Can you work these out from the drawing? Everything is in mm from the part's minimum corner. Round coordinates to 2 decimals unless told otherwise and drop trailing zeros. Order: outer loops, then holes, each group sorted by start corner. A loop starts at its lowest first (then second) coordinate and runs counter-clockwise, first axis right, second up. Notation, with made-up numbers: (89, 67.25) - (141, 67.25) arc R19 cw to (141, 72.25) - close; hole circle Ø8 at (-0.5, -7). An arc over 180 degrees is marked (long way). Write item = value, one per line.
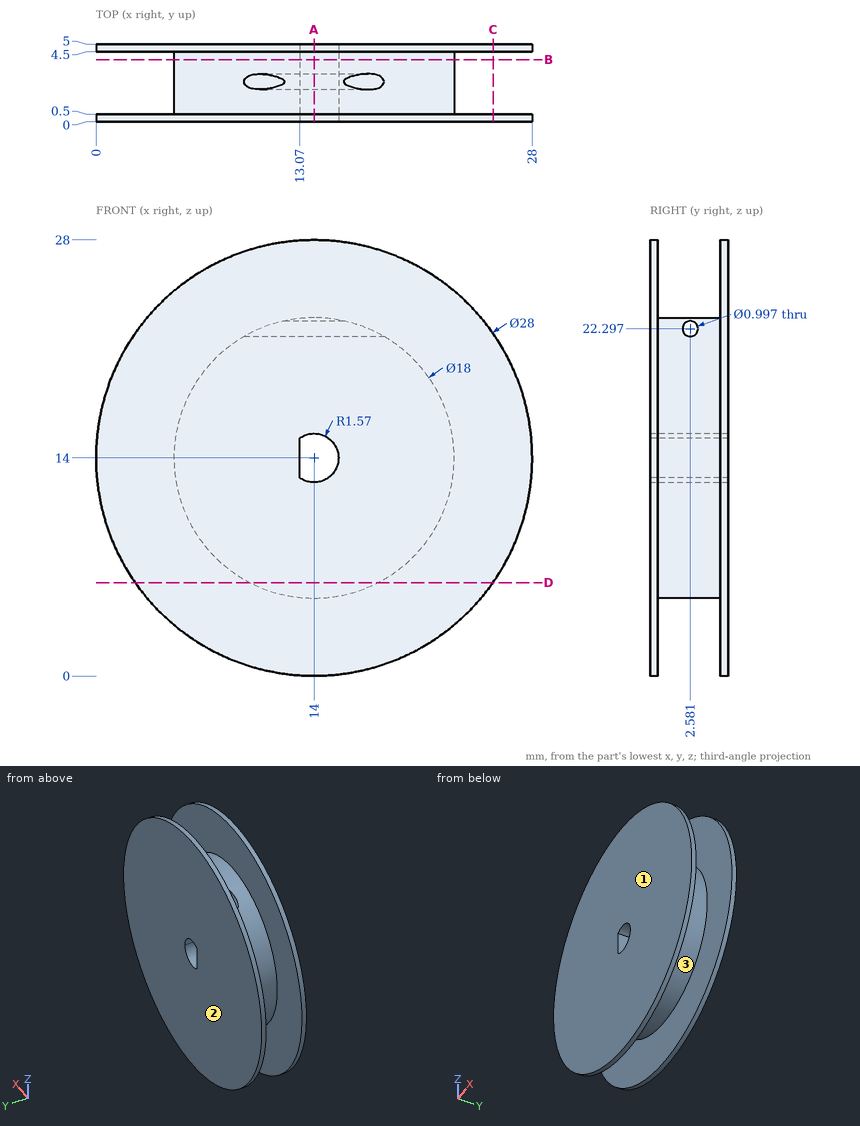
(1) Thinking about a two-plate mould opening in Y: for the marked faces 1, 2 and 3, which applies, +Y half, -Y half, draft (parallel to the pull), parting line (faces both ways), or undercut?
Computed:
face_1 = -Y half
face_2 = +Y half
face_3 = undercut
(2) If we section it at C-C (x = 25.5): Write out the boundary of the cut face in (y, z) (1 decimal).
Computed:
outline = (0, 6) - (0.5, 6) - (0.5, 22) - (0, 22) - close; (4.5, 6) - (5, 6) - (5, 22) - (4.5, 22) - close
(3) If we section it at B-B (y = 4): Write out the boundary of the cut face in (x, z) (1 decimal).
Computed:
outline = circle Ø18 at (14, 14); hole (13.1, 12.7) arc R1.6 ccw (long way) to (13.1, 15.3) - close
(4) If I drill on line 1 (Y direction, x = 9.5, z = 1.5); line 2 (X direction, y = 2.2, z = 13.5) (1 decimal); line 3 (X direction, y = 3.4, z = 13) (1 decimal), over which ranges is the centre line in solid material (lowest first)? Write a range as from..to.
Computed:
line_1 = 0..0.5, 4.5..5
line_2 = 5..13.1, 15.5..23
line_3 = 5.1..13.1, 15.2..22.9
(5) If we section it at D-D (z = 6): Write out the boundary of the cut face in (x, y).
Computed:
outline = (2.51, 0) - (25.49, 0) - (25.49, 0.5) - (18.12, 0.5) - (18.12, 4.5) - (25.49, 4.5) - (25.49, 5) - (2.51, 5) - (2.51, 4.5) - (9.88, 4.5) - (9.88, 0.5) - (2.51, 0.5) - close
(6) If we section it at A-A (x = 14): Write out the boundary of the cut face in (y, z).
Computed:
outline = (0, 0) - (0.5, 0) - (0.5, 5) - (4.5, 5) - (4.5, 0) - (5, 0) - (5, 12.43) - (0, 12.43) - close; (0, 15.57) - (5, 15.57) - (5, 28) - (4.5, 28) - (4.5, 23) - (0.5, 23) - (0.5, 28) - (0, 28) - close; hole circle Ø1 at (2.58, 22.3)
(7) Will these pins go through, and if not, where does the flat tip stop? P1, Ø1, axis at y = 3.5, z = 12, coming from the -X side; P2, Ø8, axis at x = 19.5, z = 21, coming from the -Y side; P3, Ø1.3, axis at y = 3.5, z = 14.5, coming from the +X side; P4, Ø3, axis at x = 6.5, y = 4, coming from the -Z side.
Computed:
P1 = 5.13
P2 = 0
P3 = 23
P4 = 1.39
